For this review, use the dimensioned drawing (mm, ordinates from the lowest corner) and the shaded views. A direction names the side the tool comes from. Give positions to 0.01 mm unless a question says otherwise; leave off trailing zeros. Loops run counter-clockwise (first coordinate to the right, second up) from the corner with the lowest first, then second, coordinate; pieces in that order, holes last. Notation, with made-up numbers: M 49,-11.5 L 60,-11.5 A11 cw 60,0.5 Z; hole C 14.25,41.25 d8. An arc over 180 degrees is marked long. Use a Markdown table: item, result. Add a question column.
(1) For probe 1 along X at (y, z) = (5.25, 7.25) (1 decimal); probe 2 along Y at (x, z) = (10.5, 2.25) (1 decimal); probe 3 along Y at (x, z) = (8.25, 3) (1 decimal), list the stretches that pass through material, from the lowest coordinate up.
(2) For the marked faces 4, 5, 6 and 7, list the 3-axis set-ups (+Z, -Z, +X, -X, +Y, -Y) from which the entire face can be reached by the end or side of a thin tool; tool diameter is ignored.
(3) Add section B-B, the plane z = 12. State how many separate pieces and enclosed holes the cut face has.
(4) Draft analysis for pull direction Y (two halves, no side actions). For the marked faces 1, 2 and 3, state which applies: pulls with the +Y half, pulls with the -Y half, needs draft (parallel to the pull), parting line crosses it, or undercut.
(5) Add section A-A, the plane y = 5.25. Give the boundary of the cut face in (x, z) (1 decimal).
(6) Insertion check: pin 1 Ø1 at (y, z) = (8.5, 12.5) entering from +X; pin 2 Ø3 at (y, z) = (10, 8) entering from +X; pin 3 Ø2 at (y, z) = (10.5, 5) entering from -X; pin 4 Ø5 at (x, y) = (7.5, 5) entering from +Z. Each pin has a flat end and moves straight along its axis. Give the tip position at first contact, or say it passes through.
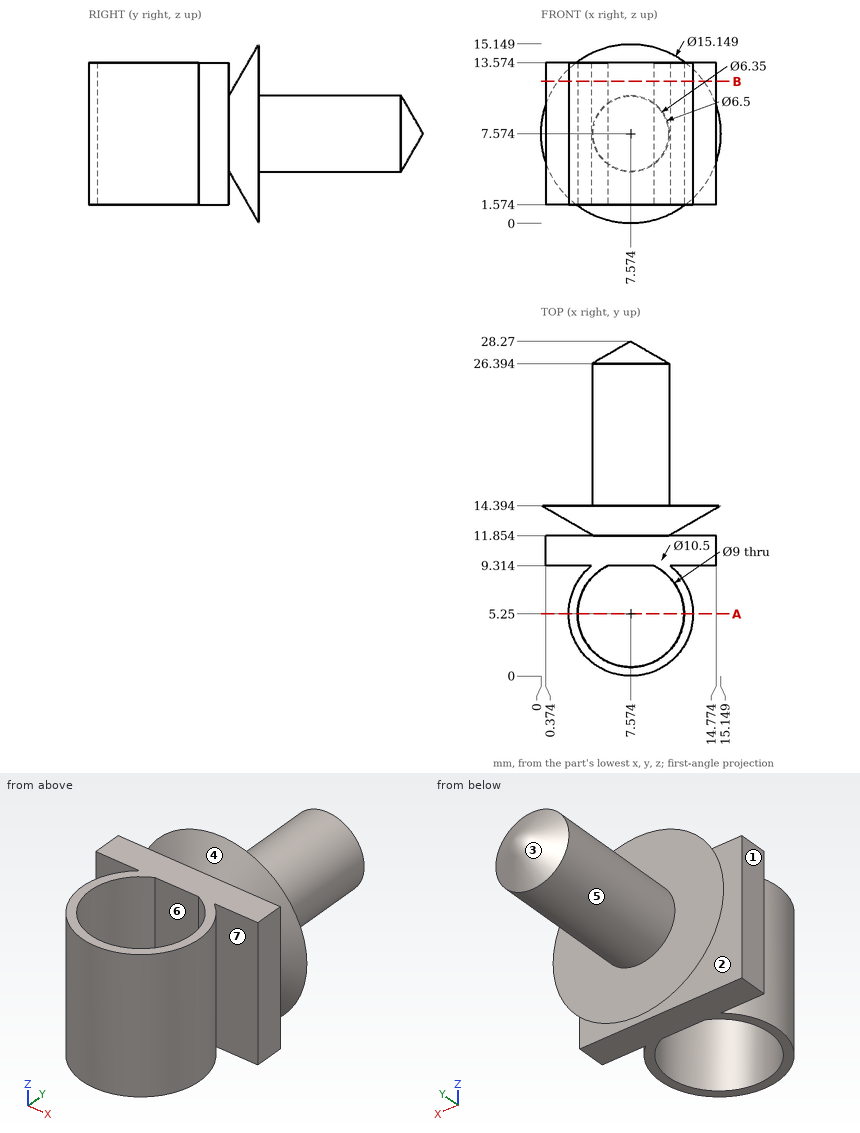
Established:
| question | item | result |
|---|---|---|
| 1 | probe 1 | 2.3 to 3.1, 12.1 to 12.8 |
| 1 | probe 2 | 0.9 to 1.8, 8.7 to 11.9, 13.5 to 14.4 |
| 1 | probe 3 | 0 to 0.8, 9.3 to 11.9, 12.7 to 14.4 |
| 2 | face 4 | none |
| 2 | face 5 | +Y |
| 2 | face 6 | +Z, -Z |
| 2 | face 7 | +Z, -Z, +X |
| 3 | separate pieces | 2 |
| 3 | enclosed holes | 1 |
| 4 | face 1 | needs draft |
| 4 | face 2 | undercut |
| 4 | face 3 | pulls with the +Y half |
| 5 | outline | M 2.3,1.6 L 3.1,1.6 L 3.1,13.6 L 2.3,13.6 Z; M 12.1,1.6 L 12.8,1.6 L 12.8,13.6 L 12.1,13.6 Z |
| 6 | pin 1 | x = 12.05 |
| 6 | pin 2 | x = 14.77 |
| 6 | pin 3 | x = 0.37 |
| 6 | pin 4 | through |
